Can you work these out from the model? Positions are in its coordinate system, mm. Face numbers are marked on the shaded views. A direction names the side the tool comes from. Round coordinates to 2 decimals unless told otherwise and drop trailing zeros. Loops run counter-clockwise (first coordinate to the right, second up) from the corner with the lowest first, then second, coordinate; pieces in that order, holes last. Notation, with made-up numbers: (67, 86.5) -> (105, 86.5) arc R29 ccw to (105, 124.5) -> close; hole circle Ø8 at (-1.5, 36.5). An arc over 180 degrees is marked (long way). Use a Markdown table: item, result.
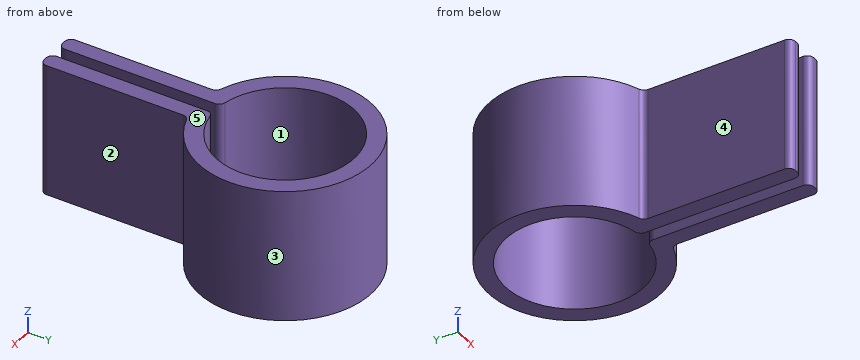
from build123d import *

# Parameters (mm, degrees)
BOSS_EXTRUDE1_DEPTH = 10


with BuildPart() as part:
    # Sketch1 → Boss-Extrude1 (new body)
    with BuildSketch(Plane.XY):
        with BuildLine():
            Line((0.478661478, -5.615355885), (0.478661478, -16.97170584))
            ThreePointArc((0.478661478, -16.97170584), (0.625108087, -17.325259231), (0.978661478, -17.47170584))
            Line((0.978661478, -17.47170584), (1.209808881, -17.47170584))
            ThreePointArc((1.209808881, -17.47170584), (1.563362272, -17.325259231), (1.709808881, -16.97170584))
            Line((1.709808881, -16.97170584), (1.709808881, -6.642043715))
            ThreePointArc((1.709808881, -6.642043715), (1.804271123, -6.349572986), (2.05196539, -6.167612021))
            ThreePointArc((2.05196539, -6.167612021), (0, 6.5), (-2.05196539, -6.167612021))
            ThreePointArc((-2.05196539, -6.167612021), (-1.804271123, -6.349572986), (-1.709808881, -6.642043715))
            Line((-1.709808881, -6.642043715), (-1.709808881, -16.97170584))
            ThreePointArc((-1.709808881, -16.97170584), (-1.563362272, -17.325259231), (-1.209808881, -17.47170584))
            Line((-1.209808881, -17.47170584), (-0.978661478, -17.47170584))
            ThreePointArc((-0.978661478, -17.47170584), (-0.625108087, -17.325259231), (-0.478661478, -16.97170584))
            Line((-0.478661478, -16.97170584), (-0.478661478, -5.615355885))
            ThreePointArc((-0.478661478, -5.615355885), (-0.595958101, -5.293582478), (-0.89281398, -5.122780807))
            ThreePointArc((-0.89281398, -5.122780807), (0, 5.2), (0.89281398, -5.122780807))
            ThreePointArc((0.89281398, -5.122780807), (0.595958101, -5.293582478), (0.478661478, -5.615355885))
        make_face()
    extrude(amount=BOSS_EXTRUDE1_DEPTH)


solid = part.part
1. I want a section at C-C (z = 5). Please give me the cut outline in (x, y), plus the area to 3 significant figures.
Answer sheet:
| item | result |
|---|---|
| outline | (-2.05, -6.17) arc R0.5 cw to (-1.71, -6.64) -> (-1.71, -16.97) arc R0.5 ccw to (-1.21, -17.47) -> (-0.98, -17.47) arc R0.5 ccw to (-0.48, -16.97) -> (-0.48, -5.62) arc R0.5 ccw to (-0.89, -5.12) arc R5.2 cw (long way) to (0.89, -5.12) arc R0.5 ccw to (0.48, -5.62) -> (0.48, -16.97) arc R0.5 ccw to (0.98, -17.47) -> (1.21, -17.47) arc R0.5 ccw to (1.71, -16.97) -> (1.71, -6.64) arc R0.5 cw to (2.05, -6.17) arc R6.5 ccw (long way) to start |
| area | 73.6 mm² |
2. I want a section at A-A (y = 0). Please give me the cut outline in (x, z), plus the area to 3 significant figures.
Answer sheet:
| item | result |
|---|---|
| outline | (-6.5, 0) -> (-5.2, 0) -> (-5.2, 10) -> (-6.5, 10) -> close; (5.2, 0) -> (6.5, 0) -> (6.5, 10) -> (5.2, 10) -> close |
| area | 26.0 mm² |
3. Will these pins go through, and if not, where does the flat tip stop? pin 1 Ø3 at (x, z) = (5, 8.5) entering from -Y; pin 2 Ø5 at (y, z) = (-12.5, 6.5) entering from +X; pin 3 Ø5 at (y, z) = (-13, 7) entering from -X.
Answer sheet:
| item | result |
|---|---|
| pin 1 | stops at y = -5.48 |
| pin 2 | stops at x = 1.71 |
| pin 3 | stops at x = -1.71 |
4. I want a section at B-B (x = -3). Please give me the cut outline in (y, z).
Answer sheet:
| item | result |
|---|---|
| outline | (-5.77, 0) -> (-4.25, 0) -> (-4.25, 10) -> (-5.77, 10) -> close; (4.25, 0) -> (5.77, 0) -> (5.77, 10) -> (4.25, 10) -> close |
5. I need wall thicknesses on line 1 (X direction, y = 0, z = 4.75); line 2 (X direction, y = -10.5, z = 5.5); line 3 (Y direction, x = -3, z = 7). Which ranges of each line are inside material? Lowest first, please.
Answer sheet:
| item | result |
|---|---|
| line 1 | x = -6.5 to -5.2, 5.2 to 6.5 |
| line 2 | x = -1.71 to -0.48, 0.48 to 1.71 |
| line 3 | y = -5.77 to -4.25, 4.25 to 5.77 |
6. If we mould it in two halves opening along Y, with no side actions, what happens to the marked faces 1, 2 and 3? For each: +Y half, -Y half, draft (parallel to the pull), parting line (faces both ways), or undercut.
Answer sheet:
| item | result |
|---|---|
| face 1 | undercut |
| face 2 | draft |
| face 3 | parting line |
7. Which directions (+Z, -Z, +X, -X, +Y, -Y) give clear straight access to the entire face, cutting with the end or side of a thin tool? Please do the marked faces 4 and 5.
Answer sheet:
| item | result |
|---|---|
| face 4 | +Z, -Z, -X, -Y |
| face 5 | +Z, +X, -X, +Y, -Y |
8. I want a section at D-D (x = 0). Please give me the cut outline in (y, z).
Answer sheet:
| item | result |
|---|---|
| outline | (5.2, 0) -> (6.5, 0) -> (6.5, 10) -> (5.2, 10) -> close |
